Build history of the part. All positions in model axes, mm. A direction names the side the tool comes from. Give positions to 0.01 mm unless a question says otherwise; leave off trailing zeros. Order: outer loops, then holes, each group sorted by start corner. A loop starts at its lowest first (then second) coordinate and runs counter-clockwise, first axis right, second up. Notation, with made-up numbers: (-32, -28) - (-27, -28) arc R33 ccw to (-27, 5) - close; hole circle Ø5 at (-14.75, 44.5). An arc over 180 degrees is marked (long way). Answer in a Markdown table with one row per item.
```python
from build123d import *

# Parameters (mm, degrees)
DODANIE_WYCI_GNI_CIE1_DEPTH = 180
SZKIC2_W                    = 10.5
SZKIC2_H                    = 20
WYTNIJ_WYCI_GNI_CIE1_DEPTH  = 183.921602059
SZKIC3_R                    = 2
WYTNIJ_WYCI_GNI_CIE2_DEPTH  = 10
SZKIC4_R                    = 2
WYTNIJ_WYCI_GNI_CIE3_DEPTH  = 10
SZKIC5_R                    = 2.5
WYTNIJ_WYCI_GNI_CIE4_DEPTH  = 10


with BuildPart() as part:
    # Szkic1 → Dodanie-wyciągnięcie1 (new body)
    with BuildSketch(Plane.XY):
        Polygon((9.75, -9.75), (9.75, -15.75), (-20.25, -15.75), (-20.25, 9.75), (-9.75, 9.75), (-9.75, -9.75), align=None)
    extrude(amount=DODANIE_WYCI_GNI_CIE1_DEPTH)

    # Szkic2 → Wytnij-wyciągnięcie1 (cut, through all)
    with BuildSketch(Plane(origin=(0, 9.75, 0), x_dir=(1, 0, 0), z_dir=(0, 1, 0))):
        with Locations((-15, -170)):
            Rectangle(SZKIC2_W, SZKIC2_H)
    wytnij_wyci_gni_cie1 = extrude(amount=-WYTNIJ_WYCI_GNI_CIE1_DEPTH, mode=Mode.SUBTRACT)

    # Lustro1: Wytnij-wyciągnięcie1 across plane
    add(wytnij_wyci_gni_cie1.mirror(Plane.XY.offset(90)), mode=Mode.SUBTRACT)

    # Szkic3 → Wytnij-wyciągnięcie2 (cut)
    with BuildSketch(Plane(origin=(0, 9.75, 0), x_dir=(1, 0, 0), z_dir=(0, 1, 0))):
        with Locations(Location((-14.75, -55, 0), (0, 0, 180))):
            Circle(SZKIC3_R)
        with Locations(Location((-14.75, -125, 0), (0, 0, 180))):
            Circle(SZKIC3_R)
    extrude(amount=-WYTNIJ_WYCI_GNI_CIE2_DEPTH, mode=Mode.SUBTRACT)

    # Szkic4 → Wytnij-wyciągnięcie3 (cut)
    with BuildSketch(Plane.XY.offset(160)):
        with Locations((-14.75, -5.25)):
            Circle(SZKIC4_R)
    wytnij_wyci_gni_cie3 = extrude(amount=-WYTNIJ_WYCI_GNI_CIE3_DEPTH, mode=Mode.SUBTRACT)

    # Lustro2: Wytnij-wyciągnięcie3 across plane
    add(wytnij_wyci_gni_cie3.mirror(Plane.XY.offset(90)), mode=Mode.SUBTRACT)

    # Szkic5 → Wytnij-wyciągnięcie4 (cut)
    with BuildSketch(Plane(origin=(0, -9.75, 0), x_dir=(1, 0, 0), z_dir=(0, 1, 0))):
        with Locations(Location((0.25, -90, 0), (0, 0, 270))):
            Circle(SZKIC5_R)
    extrude(amount=-WYTNIJ_WYCI_GNI_CIE4_DEPTH, mode=Mode.SUBTRACT)


solid = part.part
```
1. Cut at C-C on z = 90. Write the cut outline in (x, y).
Check result:
| item | result |
|---|---|
| outline | (-20.25, -15.75) - (-2.25, -15.75) - (-2.25, -9.75) - (-9.75, -9.75) - (-9.75, 9.75) - (-20.25, 9.75) - close; (2.75, -15.75) - (9.75, -15.75) - (9.75, -9.75) - (2.75, -9.75) - close |
2. Two-plate mould, pull along Z, no slides. Class faces 1 (the face through (-15.8, 4.8, 126.7)), 2 (the face through (0, -13, 0)), 3 (the face through (0, -13, 180)): +Z half, -Z half, draft (parallel to the pull), parting line (faces both ways), or undercut.
Check result:
| item | result |
|---|---|
| face 1 | undercut |
| face 2 | -Z half |
| face 3 | +Z half |
3. Drop flat-ended pins along their axis: P1, Ø1.2, axis at x = -15, z = 125, coming from the +Y side; P2, Ø10, axis at x = -1, z = 90.5, coming from the +Y side; P3, Ø1.8, axis at y = -12.5, z = 8.5, coming from the -X side. Give the stop position or say it passes through.
Check result:
| item | result |
|---|---|
| P1 | stops at y = -0.25 |
| P2 | stops at y = -9.75 |
| P3 | stops at x = -9.75 |
4. Which spindle directions (+Z, -Z, +X, -X, +Y, -Y) get a long thin tool onto all of the face, cutting with end or side? Do faces 4 (the face through (-14.49, 4.82, 56.983)), 5 (the face through (-15, -5, 30)), 6 (the face through (-9.75, 0, 89)), 7 (the face through (-15, -3, 160)). Say none if no direction does.
Check result:
| item | result |
|---|---|
| face 4 | +Y |
| face 5 | -Z |
| face 6 | +Z, -Z, +X, +Y |
| face 7 | +Z, -X, +Y, -Y |
5. Probe line 1 (Z direction, x = -14.75, y = 5.75); line 2 (X direction, y = -11.45, z = 90); line 3 (Y direction, x = -14.75, z = 157). List the from-to ranges inside material, lowest first.
Check result:
| item | result |
|---|---|
| line 1 | z = 20 to 53, 57 to 123, 127 to 160 |
| line 2 | x = -20.25 to -2.25, 2.75 to 9.75 |
| line 3 | y = -15.75 to -7.25, -3.25 to 9.75 |
6. Cut at A-A on y = -12. Write the cut outline in (x, z).
Check result:
| item | result |
|---|---|
| outline | (-20.25, 20) - (-9.75, 20) - (-9.75, 0) - (9.75, 0) - (9.75, 180) - (-9.75, 180) - (-9.75, 160) - (-20.25, 160) - close; hole circle Ø5 at (0.25, 90) |
7. Cut at D-D on z = 125. Write the cut outline in (x, y), and give its area (3 significant figures).
Check result:
| item | result |
|---|---|
| outline | (-20.25, -15.75) - (9.75, -15.75) - (9.75, -9.75) - (-9.75, -9.75) - (-9.75, 9.75) - (-12.75, 9.75) - (-12.75, -0.25) - (-16.75, -0.25) - (-16.75, 9.75) - (-20.25, 9.75) - close |
| area | 345 mm² |
8. Cut at B-B on x = -14.75. Write the cut outline in (y, z).
Check result:
| item | result |
|---|---|
| outline | (-15.75, 20) - (-7.25, 20) - (-7.25, 30) - (-3.25, 30) - (-3.25, 20) - (9.75, 20) - (9.75, 53) - (-0.25, 53) - (-0.25, 57) - (9.75, 57) - (9.75, 123) - (-0.25, 123) - (-0.25, 127) - (9.75, 127) - (9.75, 160) - (-3.25, 160) - (-3.25, 150) - (-7.25, 150) - (-7.25, 160) - (-15.75, 160) - close |
